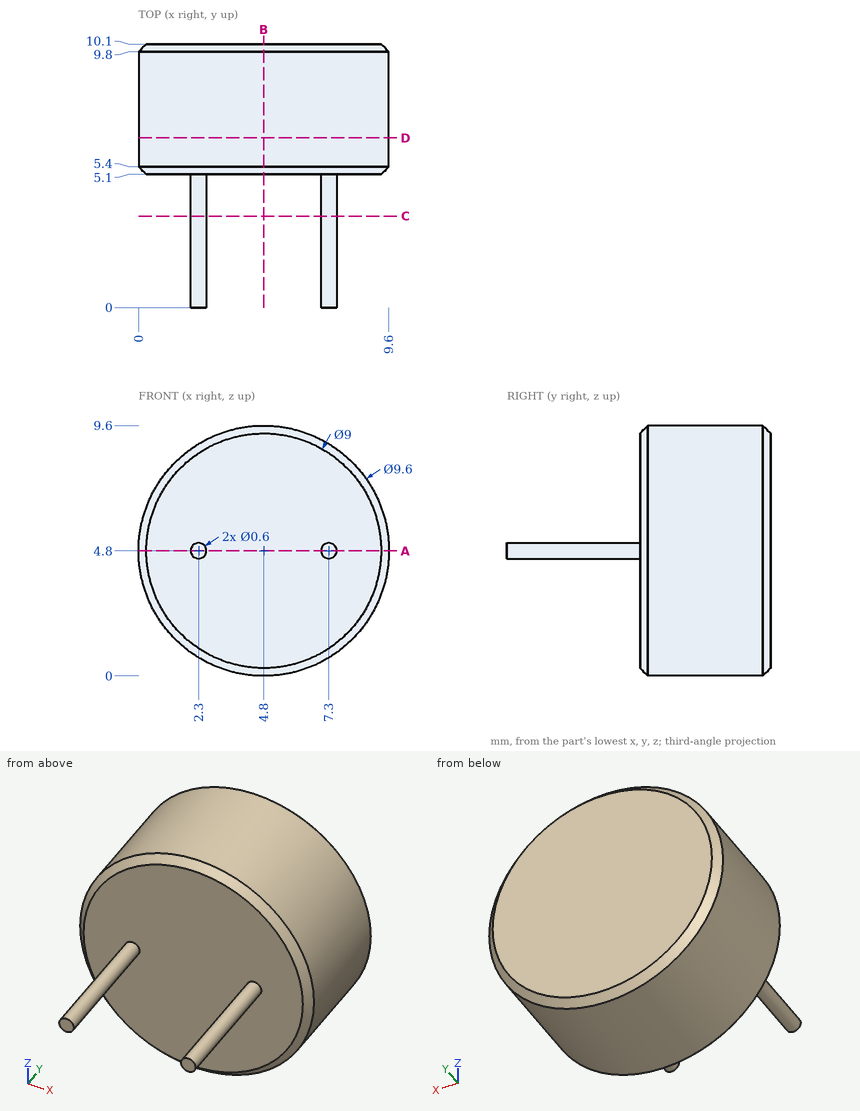
Study the drawing (mm; zero at the part's minimum x, y, z) and answer. Coordinates: 2 decimals unless noted, no trailing zeros. Write each loop counter-clockwise with the first axis right and the second up, starting at its lowest first coordinate (ties: lowest second). Pieces come first, ordered by that corner, then holes. Notation, with made-up numbers: (44.5, 13.5) - (71.5, 13.5) arc R28 cw to (71.5, 42.5) - close; hole circle Ø3 at (-17, -11). An arc over 180 degrees is marked (long way). Answer as a JSON object with one key per item and string values. Group by question number.
1. A cutting plane is placed at D-D (y = 6.5). Determine the outline of the cut face in (x, z).
2. Consider L1, parallel to Y at x = 1.75, z = 2.25; L2, parallel to Z at x = 4.5, y = 9.5; L3, parallel to Z at x = 1, y = 6.25. Determine where each line is inside the solid, lowest interval first. Write a range as [from, to].
3. Each of these flat-tipped pins is pushed along its axis until it touches: P1, Ø4, axis at x = 2, y = 8, coming from the -Z side; P2, Ø1, axis at x = 3, z = 4, coming from the -Y side; P3, Ø1, axis at y = 8.5, z = 5.5, coming from the +X side. Where does it stop, or does it pass through?
4. A cutting plane is placed at B-B (x = 4.8). Determine the outline of the cut face in (y, z).
5. A cutting plane is placed at C-C (y = 3.5). Determine the outline of the cut face in (x, z).
6. A cutting plane is placed at A-A (z = 4.8). Determine the outline of the cut face in (x, y), plus the area to 3 significant figures.
Worked out:
{
 "1": {"outline": "circle Ø9.6 at (4.8, 4.8)"},
 "2": {"L1": "y = [5.1, 10.1]", "L2": "z = [0.01, 9.59]", "L3": "z = [1.87, 7.73]"},
 "3": {"P1": "stops at z = 0.07", "P2": "stops at y = 5.1", "P3": "stops at x = 9.6"},
 "4": {"outline": "(5.1, 0.3) - (5.4, 0) - (9.8, 0) - (10.1, 0.3) - (10.1, 9.3) - (9.8, 9.6) - (5.4, 9.6) - (5.1, 9.3) - close"},
 "5": {"outline": "circle Ø0.6 at (2.3, 4.8); circle Ø0.6 at (7.3, 4.8)"},
 "6": {"outline": "(0, 5.4) - (0.3, 5.1) - (2, 5.1) - (2, 0) - (2.6, 0) - (2.6, 5.1) - (7, 5.1) - (7, 0) - (7.6, 0) - (7.6, 5.1) - (9.3, 5.1) - (9.6, 5.4) - (9.6, 9.8) - (9.3, 10.1) - (0.3, 10.1) - (0, 9.8) - close", "area": "53.9 mm²"}
}
